Geometry: final body of the model. Coordinates: model frame, mm. Round coordinates to 2 decimals unless told otherwise and drop trailing zeros. Order: outer loops, then holes, each group sorted by start corner. A loop starts at its lowest first (then second) coordinate and runs counter-clockwise, first axis right, second up. Notation, with made-up numbers: M -24,-30.5 L 4,-30.5 A31 ccw 4,8.5 Z; hole C 72,6 d9. An arc over 180 degrees is marked long. Return JSON: item names as keys, results as strings. Group by question number.
Q1. Cut plane B-B on x = -2. Output: boundary loops of the cut face in (y, z), and give its area (3 significant figures).
Q2. Ray query, probe 1 along Y at (x, z) = (-0.25, -0.65); probe 2 along Z at (x, y) = (1.5, 11.75); probe 3 along X at (y, z) = (11.4, -0.6). Return the intervals inside material, ascending.
Q3. Contact query for a flat-ended pin moving along its axis: pin 1 (1 mm diameter, centred on x = -2.5, y = 10, fed in from +Z). Output: stop coordinate, or through.
Q4. Cut plane A-A on y = 10.15. Output: boundary loops of the cut face in (x, z), and give its area (3 significant figures).
```python
from build123d import *

# Parameters (mm, degrees)
EXTRUDE_1_DEPTH     = 20
SKETCH_4_W          = 39.68109217
SKETCH_4_H          = 19.592945183
CUT_EXTRUDE_1_DEPTH = 20
SKETCH_7_W          = 132.193091595
SKETCH_7_H          = 30.201739996
CUT_EXTRUDE_2_DEPTH = 20
SCALE_1_SCALE       = 0.2


with BuildPart() as part:
    # 草圖1 → 填料-伸長1 (new body)
    with BuildSketch(Plane(origin=(0, 0, 0), x_dir=(1, 0, 0), z_dir=(0, 1, 0))):
        Polygon((15, -5), (-10, -10), (-15, -10), (-15, 10), (15, 10), align=None)
    extrude(amount=EXTRUDE_1_DEPTH)

    # 草圖4 → 除料-伸長1 (cut)
    with BuildSketch(Plane(origin=(6.101694915, 10.169491525, 10.169491525), x_dir=(0.920574618, -0.276172385, -0.276172385), z_dir=(0.390566733, 0.650944555, 0.650944555))):
        with Locations((1.579314275, 10.72678571)):
            Rectangle(SKETCH_4_W, SKETCH_4_H)
    extrude(amount=CUT_EXTRUDE_1_DEPTH, mode=Mode.SUBTRACT)

    # 草圖7 → 除料-伸長2 (cut)
    with BuildSketch(Plane(origin=(1.016949153, -1.694915254, 1.694915254), x_dir=(-0.920574618, -0.276172385, 0.276172385), z_dir=(-0.390566733, 0.650944555, -0.650944555))):
        with Locations((9.754035329, 10.9182289)):
            Rectangle(SKETCH_7_W, SKETCH_7_H)
    extrude(amount=-CUT_EXTRUDE_2_DEPTH, mode=Mode.SUBTRACT)


with BuildPart() as part_1:
    # 縮放比例1: scaled about (-1.575630252, 10, -1.365546218)
    add(part.part.scale(SCALE_1_SCALE).moved(Location((-1.260504202, 8, -1.092436974))))


solid = part_1.part
```
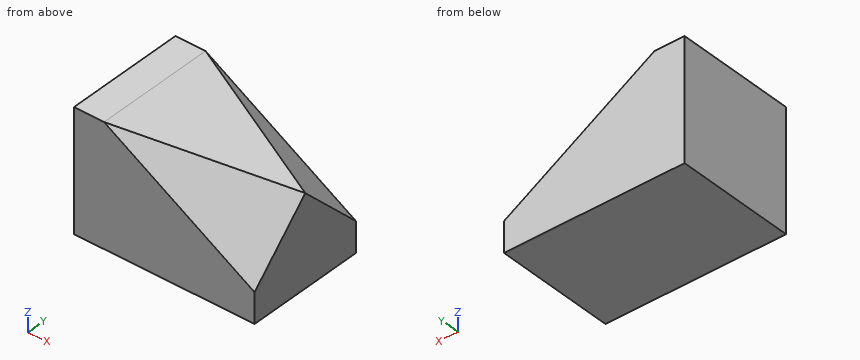
Result sheet:
{
 "1": {"outline": "M 8,-3.09 L 12,-3.09 L 12,0.15 L 11.5,0.66 L 8.5,0.66 L 8,0.15 Z", "area": "14.7 mm²"},
 "2": {"probe 1": "y = 8.25 to 11.75", "probe 2": "z = -3.09 to -1.7", "probe 3": "x = -4.26 to 0.25"},
 "3": {"pin 1": "stops at z = 0.86"},
 "4": {"outline": "M -4.26,-3.09 L 1.74,-3.09 L 1.74,-0.24 L 1.36,-0.02 L -3.26,0.91 L -4.26,0.91 Z", "area": "21.5 mm²"}
}
